```python
from build123d import *

# Parameters (mm, degrees)
SKETCH1_W           = 38.1
SKETCH1_H           = 25.415165138
BOSS_EXTRUDE1_DEPTH = 3.0734
SKETCH2_W           = 28.174522189
SKETCH2_H           = 63.5
BOSS_EXTRUDE2_DEPTH = 3.048
SKETCH3_W           = 2.759357051
SKETCH3_H           = 63.5
CUT_EXTRUDE1_DEPTH  = 3.048
FILLET1_R           = 3.81
SKETCH4_R           = 5.185736545
SKETCH4_R_2         = 5.105364429
SKETCH4_R_3         = 5.151648863
CUT_EXTRUDE2_DEPTH  = 3.048
SKETCH5_R           = 5.027262634
SKETCH5_R_2         = 4.974374785
CUT_EXTRUDE3_DEPTH  = 3.556


with BuildPart() as part:
    # Sketch1 → Boss-Extrude1 (new body)
    with BuildSketch(Plane(origin=(0, 0, 0), x_dir=(1, 0, 0), z_dir=(0, 1, 0))):
        with Locations((-19.05, 12.707582569)):
            Rectangle(SKETCH1_W, SKETCH1_H)
    extrude(amount=BOSS_EXTRUDE1_DEPTH)

    # Sketch2 → Boss-Extrude2 (add)
    with BuildSketch(Plane.ZY.offset(38.1)):
        with Locations((-11.327904044, 34.8234)):
            Rectangle(SKETCH2_W, SKETCH2_H)
    extrude(amount=-BOSS_EXTRUDE2_DEPTH)

    # Sketch3 → Cut-Extrude1 (cut)
    with BuildSketch(Plane(origin=(-35.052, 0, 0), x_dir=(0, 0, -1), z_dir=(1, 0, 0))):
        with Locations((-1.379678526, 34.8234)):
            Rectangle(SKETCH3_W, SKETCH3_H)
    extrude(amount=-CUT_EXTRUDE1_DEPTH, mode=Mode.SUBTRACT)

    # Fillet1
    fillet1_edges = [part.edges().sort_by_distance(p)[0] for p in [
        (-38.1, 0, -12.707582569),
    ]]
    fillet(fillet1_edges, radius=FILLET1_R)

    # Sketch4 → Cut-Extrude2 (cut)
    with BuildSketch(Plane(origin=(-35.052, 0, 0), x_dir=(0, 0, -1), z_dir=(1, 0, 0))):
        with Locations((12.7, 57.15)):
            Circle(SKETCH4_R)
        with Locations((12.7, 43.18)):
            Circle(SKETCH4_R_2)
        with Locations((12.7, 29.21)):
            Circle(SKETCH4_R_3)
    extrude(amount=-CUT_EXTRUDE2_DEPTH, mode=Mode.SUBTRACT)

    # Sketch5 → Cut-Extrude3 (cut)
    with BuildSketch(Plane(origin=(0, 0, 0), x_dir=(-1, 0, 0), z_dir=(0, -1, 0))):
        with Locations(Location((22.86, 12.7, 0), (0, 0, 90))):
            Circle(SKETCH5_R)
        with Locations(Location((8.89, 12.7, 0), (0, 0, 90))):
            Circle(SKETCH5_R_2)
    extrude(amount=-CUT_EXTRUDE3_DEPTH, mode=Mode.SUBTRACT)


solid = part.part
```
Geometry check sheet. Reference: the model listing, model coordinates, mm. A direction names the side the tool comes from. Coordinates: 2 decimals unless noted, no trailing zeros. Write each loop counter-clockwise with the first axis right and the second up, starting at its lowest first coordinate (ties: lowest second). Pieces come first, ordered by that corner, then holes. Notation, with made-up numbers: M 84,-27 L 129,-27 A7 cw 129,-15 Z; hole C 18,76 d1. An arc over 180 degrees is marked long. One line per item, written item: value. Start each with the question number.
(1) Sectioned sample at A-A, the plane z = -12.7. Enter the section's corners in (x, y), and give its area (3 significant figures).
(2) Tool access check on faces 1 (the face through (-36.55, 55.16, -17.49)), 2 (the face through (-18, 3.073, -10)). Record the directions out of +Z, -Z, +X, -X, +Y, -Y that give a thin tool (end or side, any length) a straight path to the whole face; none if there is none.
(3) Sectioned sample at C-C, the plane x = -22.86. Enter the section's corners in (y, z), and give its area (3 significant figures).
(4) Sectioned sample at D-D, the plane z = -6.25. Enter the section's corners in (x, y), and give its area (3 significant figures).
(5) Depth check by flat-ended pin: pin 1 (3 mm diameter, centred on y = 20, z = -10, fed in from +X). Enter the tip coordinate at first touch or a pass-through.
(6) Release check for a two-part mould opening along X. For faces 3 (the face through (0, 2, -13)), 4 (the face through (-36.555, 38.196, -11.593)), 5 (the face through (-17.876, 1.515, -12.046)) record: released by +X, released by -X, zero draft, split by the parting line, or undercut.
(7) Sectioned sample at B-B, the plane y = 43.18. Enter the section's corners in (x, z), and give its area (3 significant figures).
(8) Scan lines: line 1 along X through (y, z) = (1.75, -12.7); line 2 along X through (y, z) = (10, -3.5); line 3 along Y through (x, z) = (-29.5, -23.5). Record each from-to range of solid material in increasing order. Write a range as [from, to].
Filled sheet:
1. outline: M -38.1,3.81 A3.81 ccw -34.29,0 L -27.89,0 L -27.89,3.07 L -35.05,3.07 L -35.05,24.06 L -38.1,24.06 Z; M -38.1,34.36 L -35.05,34.36 L -35.05,38.07 L -38.1,38.07 Z; M -38.1,48.29 L -35.05,48.29 L -35.05,51.96 L -38.1,51.96 Z; M -38.1,62.34 L -35.05,62.34 L -35.05,66.57 L -38.1,66.57 Z; M -17.83,0 L -13.86,0 L -13.86,3.07 L -17.83,3.07 Z; M -3.92,0 L 0,0 L 0,3.07 L -3.92,3.07 Z
1. area: 152 mm²
2. face 1: +X, -X
2. face 2: +Z, -Z, +X, +Y
3. outline: M 0,-25.42 L 3.07,-25.42 L 3.07,-17.73 L 0,-17.73 Z; M 0,-7.67 L 3.07,-7.67 L 3.07,0 L 0,0 Z
3. area: 47.2 mm²
4. outline: M -38.1,3.81 A3.81 ccw -34.29,0 L 0,0 L 0,3.07 L -35.05,3.07 L -35.05,66.57 L -38.1,66.57 Z
4. area: 308 mm²
5. pin 1: x = -35.05
6. face 3: released by +X
6. face 4: zero draft
6. face 5: undercut
7. outline: M -38.1,-25.42 L -35.05,-25.42 L -35.05,-17.81 L -38.1,-17.81 Z; M -38.1,-7.59 L -35.05,-7.59 L -35.05,0 L -38.1,0 Z
7. area: 46.3 mm²
8. line 1: [-37.5, -27.89], [-17.83, -13.86], [-3.92, 0]
8. line 2: [-38.1, -35.05]
8. line 3: [0, 3.07]
